from build123d import *

# Parameters (mm, degrees)
ESQUISSE1_W                   = 30
ESQUISSE1_H                   = 40
BOSS_EXTRU_1_DEPTH            = 14
ESQUISSE3_R                   = 3.15
ENL_V_MAT_EXTRU_1_DEPTH       = 30
ESQUISSE4_W                   = 15
ESQUISSE4_H                   = 22
ENL_V_MAT_EXTRU_2_DEPTH       = 10.25
ENL_V_MAT_EXTRU_3_DEPTH       = 4.75
ENL_V_MAT_EXTRU_4_DEPTH       = 10.25
ESQUISSE7_R                   = 1.75
ENL_V_MAT_EXTRU_5_DEPTH       = 15
ENL_V_START                   = -40
ESQUISSE9_W                   = 30
ESQUISSE9_H                   = 1
ENL_V_MAT_EXTRU_9_DEPTH       = 40
ENL_V_START_2                 = -13
ESQUISSE11_W                  = 30
ESQUISSE11_H                  = 9
ENL_V_MAT_EXTRU_10_DEPTH      = 13
ESQUISSE12_W                  = 15
ESQUISSE12_H                  = 13
BOSS_EXTRU_2_DEPTH            = 10
ESQUISSE13_R                  = 1.75
ENL_V_MAT_EXTRU_11_DEPTH      = 12
CHANFREIN1_SIZE               = 4
ESQUISSE14_W                  = 3
ESQUISSE14_H                  = 31
ENL_V_MAT_EXTRU_12_DEPTH      = 1
ENL_V_MAT_EXTRU_12_DEPTH_BACK = 14
CONG_1_R                      = 3


with BuildPart() as part:
    # Esquisse1 → Boss.-Extru.1 (new body)
    with BuildSketch(Plane.XY):
        with Locations((15, 20)):
            Rectangle(ESQUISSE1_W, ESQUISSE1_H)
    extrude(amount=BOSS_EXTRU_1_DEPTH)

    # Esquisse3 → Enlèv. mat.-Extru.1 (cut)
    with BuildSketch(Plane(origin=(0, 40, 0), x_dir=(1, 0, 0), z_dir=(0, 1, 0))):
        with Locations((24, -7)):
            Circle(ESQUISSE3_R)
    extrude(amount=-ENL_V_MAT_EXTRU_1_DEPTH, mode=Mode.SUBTRACT)

    # Esquisse4 → Enlèv. mat.-Extru.2 (cut)
    with BuildSketch(Plane.XY.offset(14)):
        with Locations((7.5, 24)):
            Rectangle(ESQUISSE4_W, ESQUISSE4_H)
    extrude(amount=-ENL_V_MAT_EXTRU_2_DEPTH, mode=Mode.SUBTRACT)

    # Esquisse5 → Enlèv. mat.-Extru.3 (cut, through all)
    with BuildSketch(Plane.XY.offset(3.75)):
        with BuildLine():
            Line((6, 30.6), (14, 30.6))
            ThreePointArc((14, 30.6), (15.6, 29), (14, 27.4))
            Line((14, 27.4), (6, 27.4))
            ThreePointArc((6, 27.4), (4.4, 29), (6, 30.6))
        make_face()
        with BuildLine():
            Line((6, 17.4), (14, 17.4))
            ThreePointArc((14, 17.4), (15.6, 19), (14, 20.6))
            Line((14, 20.6), (6, 20.6))
            ThreePointArc((6, 20.6), (4.4, 19), (6, 17.4))
        make_face()
    extrude(amount=-ENL_V_MAT_EXTRU_3_DEPTH, mode=Mode.SUBTRACT)

    # Esquisse6 → Enlèv. mat.-Extru.4 (cut)
    with BuildSketch(Plane.XY.offset(14)):
        Polygon((15, 35), (18, 35), (23, 26.339745962), (23, 13), (15, 13), align=None)
    extrude(amount=-ENL_V_MAT_EXTRU_4_DEPTH, mode=Mode.SUBTRACT)

    # Esquisse7 → Enlèv. mat.-Extru.5 (cut, through all)
    with BuildSketch(Plane.XY.offset(14)):
        with Locations((5, 6.5)):
            Circle(ESQUISSE7_R)
        with Locations((25, 6.5)):
            Circle(ESQUISSE7_R)
    extrude(amount=-ENL_V_MAT_EXTRU_5_DEPTH, mode=Mode.SUBTRACT)

    # Esquisse9 → Enlèv. mat.-Extru.9 (cut)
    with BuildSketch(Plane(origin=(0, 40, 0), x_dir=(1, 0, 0), z_dir=(0, 1, 0)).offset(ENL_V_START)):
        with Locations((15, -13.5)):
            Rectangle(ESQUISSE9_W, ESQUISSE9_H)
    extrude(amount=ENL_V_MAT_EXTRU_9_DEPTH, mode=Mode.SUBTRACT)

    # Esquisse11 → Enlèv. mat.-Extru.10 (cut)
    with BuildSketch(Plane.XY.offset(13).offset(ENL_V_START_2)):
        with Locations((15, 4.5)):
            Rectangle(ESQUISSE11_W, ESQUISSE11_H)
    extrude(amount=ENL_V_MAT_EXTRU_10_DEPTH, mode=Mode.SUBTRACT)

    # Esquisse12 → Boss.-Extru.2 (add)
    with BuildSketch(Plane(origin=(0, 40, 0), x_dir=(1, 0, 0), z_dir=(0, 1, 0))):
        with Locations((37.5, -6.5)):
            Rectangle(ESQUISSE12_W, ESQUISSE12_H)
    extrude(amount=-BOSS_EXTRU_2_DEPTH)

    # Esquisse13 → Enlèv. mat.-Extru.11 (cut)
    with BuildSketch(Plane(origin=(0, 40, 0), x_dir=(1, 0, 0), z_dir=(0, 1, 0))):
        with Locations((40, -7)):
            Circle(ESQUISSE13_R)
        with Locations((8, -7)):
            Circle(ESQUISSE13_R)
    extrude(amount=-ENL_V_MAT_EXTRU_11_DEPTH, mode=Mode.SUBTRACT)

    # Chanfrein1
    chanfrein1_edges = [part.edges().sort_by_distance(p)[0] for p in [
        (30, 30, 6.5),
    ]]
    chamfer(chanfrein1_edges, length=CHANFREIN1_SIZE)

    # Esquisse14 → Enlèv. mat.-Extru.12 (cut, two sides)
    with BuildSketch(Plane.XY.offset(13)) as enl_v_mat_extru_12_sk:
        with Locations((1.5, 24.5)):
            Rectangle(ESQUISSE14_W, ESQUISSE14_H)
    extrude(amount=ENL_V_MAT_EXTRU_12_DEPTH, mode=Mode.SUBTRACT)
    extrude(enl_v_mat_extru_12_sk.sketch, amount=-ENL_V_MAT_EXTRU_12_DEPTH_BACK, mode=Mode.SUBTRACT)

    # Congé1
    cong_1_edges = [part.edges().sort_by_distance(p)[0] for p in [
        (30, 9, 6.5),
        (45, 30, 6.5),
        (45, 40, 6.5),
        (3, 9, 6.5),
        (3, 40, 6.5),
    ]]
    fillet(cong_1_edges, radius=CONG_1_R)


solid = part.part
For this review, take the finished solid that the model builds, in its own axes (mm). A direction names the side the tool comes from. Round coordinates to 2 decimals unless told otherwise and drop trailing zeros. Write each loop counter-clockwise with the first axis right and the second up, starting at its lowest first coordinate (ties: lowest second). Pieces come first, ordered by that corner, then holes. Notation, with made-up numbers: (71, 3) - (88, 3) arc R22 ccw to (88, 41) - close; hole circle Ø6 at (7.5, -36). An arc over 180 degrees is marked (long way). Write item = value, one per line. Start each with the question number.
1. Consider section C-C on x = 40. State the section outline as (y, z) points, plus the area to 3 significant figures.
2. Draft analysis for pull direction Y (two halves, no side actions). For faces 1 (the face through (44.1, 39.14, 6.41)), 2 (the face through (4.4, 29, 1.9)), 3 (the face through (26.91, 25.21, 8.21)), state which applies: released by +Y, released by -Y, zero draft, split by the parting line, or undercut.
3. Wall thickness on L1, parallel to X at y = 29, z = 3.5; L2, parallel to Z at x = 24, y = 25; L3, parallel to Y at x = 10.5, z = 1.75: over which ranges is each line inside the solid? List them lowest first.
4. Consider section B-B on y = 36. State the section outline as (x, z) points, plus the area to 3 significant figures.
5. Consider section A-A on x = 10.5. State the section outline as (y, z) points.
6. For faces 4 (the face through (8.81, 37.53, 8.55)), 5 (the face through (15.6, 19, 1.9)), 6 (the face through (23, 20, 12)), list the 3-axis set-ups (+Z, -Z, +X, -X, +Y, -Y) from which the entire face can be reached by the end or side of a thin tool; tool diameter is ignored.
7. For pin 1 Ø5 at (x, z) = (31.5, 3.5) entering from -Y; pin 2 Ø8 at (x, y) = (13, 25.5) entering from +Z; pin 3 Ø8 at (x, y) = (34.5, 13.5) entering from +Z; pin 4 Ø5.5 at (x, z) = (8, 7) entering from +Y, all flat-tipped, find the tip position at first contact; note any pin that passes through.
8. Consider section D-D on y = 19. State the section outline as (x, z) points.
Evaluation:
q1.outline = (30, 0) - (40, 0) - (40, 5.25) - (30, 5.25) - close; (30, 8.75) - (40, 8.75) - (40, 13) - (30, 13) - close
q1.area = 95.0 mm2
q2.face_1 = released by +Y
q2.face_2 = undercut
q2.face_3 = zero draft
q3.L1 = 3 to 4.4, 15.6 to 33
q3.L2 = 0 to 3.85, 10.15 to 13
q3.L3 = 9 to 17.4, 20.6 to 27.4, 30.6 to 40
q4.outline = (3, 0) - (45, 0) - (45, 13) - (3, 13) - close; hole circle Ø3.5 at (8, 7); hole circle Ø6.3 at (24, 7); hole circle Ø3.5 at (40, 7)
q4.area = 496 mm2
q5.outline = (9, 0) - (17.4, 0) - (17.4, 3.75) - (13, 3.75) - (13, 13) - (9, 13) - close; (20.6, 0) - (27.4, 0) - (27.4, 3.75) - (20.6, 3.75) - close; (30.6, 0) - (40, 0) - (40, 13) - (35, 13) - (35, 3.75) - (30.6, 3.75) - close
q6.face_4 = +Y
q6.face_5 = +Z, -Z
q6.face_6 = +Z, -X
q7.pin_1 = 9.76
q7.pin_2 = 3.75
q7.pin_3 = through
q7.pin_4 = 40
q8.outline = (3, 0) - (4.4, 0) - (4.4, 3.75) - (3, 3.75) - close; (15.6, 0) - (30, 0) - (30, 13) - (23, 13) - (23, 9.99) arc R3.15 cw (long way) to (23, 4.01) - (23, 3.75) - (15.6, 3.75) - close
